CAD build for the part. Positions are in the model's coordinates, mm. Face numbers are marked on the shaded views. Coordinates: 2 decimals unless noted, no trailing zeros. Write each loop counter-clockwise with the first axis right and the second up, starting at its lowest first coordinate (ties: lowest second). Pieces come first, ordered by that corner, then holes.
```python
from build123d import *

# Parameters (mm, degrees)
SKETCH1_W                   = 57.15
SKETCH1_H                   = 25.4
BOSS_EXTRUDE1_DEPTH         = 53.975
F_1_4_0_25_DIAMETER_HOLE1_D = 6.35
F_3_8_CLEARANCE_HOLE1_D     = 9.8044


with BuildPart() as part:
    # Sketch1 → Boss-Extrude1 (new, symmetric)
    with BuildSketch(Plane(origin=(0, 0, 0), x_dir=(1, 0, 0), z_dir=(0, 1, 0))):
        Rectangle(SKETCH1_W, SKETCH1_H)
    extrude(amount=BOSS_EXTRUDE1_DEPTH, both=True)

    # 1/4 (0.25) Diameter Hole1 (through all)
    with Locations(Plane(origin=(28.575, 0, 0), x_dir=(0, 0, -1), z_dir=(1, 0, 0))):
        with Locations((0, -34.925), (0, 34.925)):
            Hole(F_1_4_0_25_DIAMETER_HOLE1_D / 2)

    # 3/8 Clearance Hole1 (through all)
    with Locations(Plane.XY.offset(12.7)):
        with Locations((0, -44.45), (0, 25.4)):
            Hole(F_3_8_CLEARANCE_HOLE1_D / 2)


solid = part.part
```
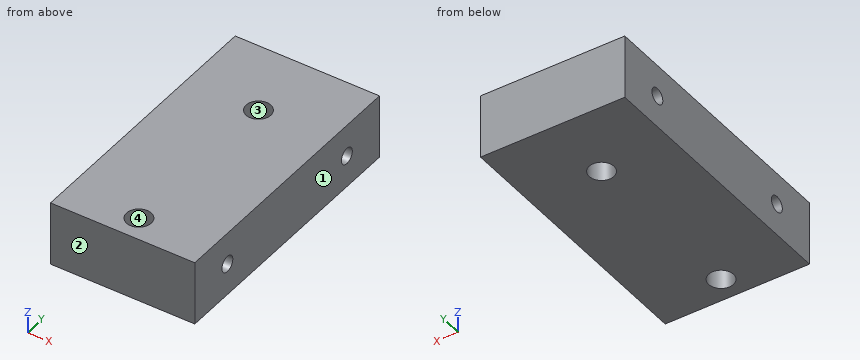
Item 1: Saw through at D-D, the plane z = -5. Write the cut outline in (x, y) (3 decimals), and give its area (3 significant figures).
Item 2: Saw through at B-B, the plane y = 25.4. Write the cut outline in (x, z) (3 decimals).
Item 3: Saw through at A-A, the plane z = 0. Write the cut outline in (x, y) (3 decimals), and give its area (3 significant figures).
Item 4: Flat gauge pins, fed straight in: pin 1 Ø12.5 at (x, y) = (0, 25.4) entering from +Z; pin 2 Ø5.5 at (y, z) = (-34.925, 0) entering from +X. Where does each tip first touch, or does it go through?
Item 5: Wall check: line 1 along Y through (x, z) = (0, 0.25) (3 decimals); line 2 along Y through (x, z) = (-16.5, 0) (3 decimals); line 3 along Y through (x, z) = (0, -5) (3 decimals). Give the ranges that are in metal, low to high.
Item 6: Two-plate mould, pull along X, no slides. Class the marked faces 1, 2, 3 and 4: +X half, -X half, draft (parallel to the pull), parting line (faces both ways), or undercut.
Item 7: Saw through at C-C, the plane x = 0. Write the cut outline in (y, z) (3 decimals), and give its area (3 significant figures).
Working result:
1. outline: (-28.575, -53.975) - (28.575, -53.975) - (28.575, 53.975) - (-28.575, 53.975) - close; hole circle Ø9.804 at (0, -44.45); hole circle Ø9.804 at (0, 25.4)
1. area: 6,020 mm2
2. outline: (-28.575, -12.7) - (-4.902, -12.7) - (-4.902, 12.7) - (-28.575, 12.7) - close; (4.902, -12.7) - (28.575, -12.7) - (28.575, 12.7) - (4.902, 12.7) - close
3. outline: (-28.575, -53.975) - (28.575, -53.975) - (28.575, -38.1) - (-28.575, -38.1) - close; (-28.575, -31.75) - (28.575, -31.75) - (28.575, 31.75) - (-28.575, 31.75) - close; (-28.575, 38.1) - (28.575, 38.1) - (28.575, 53.975) - (-28.575, 53.975) - close; hole circle Ø9.804 at (0, -44.45); hole circle Ø9.804 at (0, 25.4)
3. area: 5,290 mm2
4. pin 1: stops at z = 12.7
4. pin 2: passes through
5. line 1: y = -53.975 to -49.352, -39.548 to -38.09, -31.76 to 20.498, 30.302 to 31.76, 38.09 to 53.975
5. line 2: y = -53.975 to -38.1, -31.75 to 31.75, 38.1 to 53.975
5. line 3: y = -53.975 to -49.352, -39.548 to 20.498, 30.302 to 53.975
6. face 1: +X half
6. face 2: draft
6. face 3: undercut
6. face 4: undercut
7. outline: (-53.975, -12.7) - (-49.352, -12.7) - (-49.352, 12.7) - (-53.975, 12.7) - close; (-39.548, -12.7) - (20.498, -12.7) - (20.498, 12.7) - (-39.548, 12.7) - close; (30.302, -12.7) - (53.975, -12.7) - (53.975, 12.7) - (30.302, 12.7) - close; hole circle Ø6.35 at (-34.925, 0); hole circle Ø6.35 at (34.925, 0)
7. area: 2,180 mm2
